Source: CAD feature listing. Evaluate the final solid. Frame: model axes, mm. A direction names the side the tool comes from. Round coordinates to 2 decimals unless told otherwise and drop trailing zeros. Write each loop counter-clockwise with the first axis right and the second up, starting at its lowest first coordinate (ties: lowest second). Pieces come first, ordered by that corner, then holes. Notation, with made-up numbers: M -33.75,41 L -5.75,41 A17 cw -5.75,58 Z; hole C -35,-25 d3. An arc over 180 degrees is marked long. Answer in a Markdown table with one row per item.
from build123d import *

# Parameters (mm, degrees)
CHAMFER_1_SIZE           = 2
CHAMFER_2_SIZE           = 1
PATTERN_CIRCULAR_1_COUNT = 6


with BuildPart() as part:
    # Эскиз1 → Повернуть1 (revolve)
    with BuildSketch(Plane.XY, mode=Mode.PRIVATE) as revolve_1_sk:
        Polygon((-118.03030303, 150), (11.96969697, 150), (11.96969697, 160), (-93.03030303, 160), (-93.03030303, 190), (-118.03030303, 190), align=None)
    revolve(revolve_1_sk.sketch.rotate(Axis((-311.484848485, 0, 0), (1, 0, 0)), 90), axis=Axis((-311.484848485, 0, 0), (1, 0, 0)))

    # Фаска1
    chamfer_1_edges = [part.edges().sort_by_distance(p)[0] for p in [
        (-93.03030303, 0, -190),
    ]]
    chamfer(chamfer_1_edges, length=CHAMFER_1_SIZE)

    # Фаска2
    chamfer_2_edges = [part.edges().sort_by_distance(p)[0] for p in [
        (-118.03030303, 0, -150),
    ]]
    chamfer(chamfer_2_edges, length=CHAMFER_2_SIZE)

    # Эскиз6 → Отверстие обработанное метчиком M121 (revolve, cut)
    with BuildSketch(Plane(origin=(-118.03030303, 172.5, 0), x_dir=(0, 0, 1), z_dir=(0, 1, 0))):
        Polygon((0, 0), (0, 35.814389157), (5.1, 32.75), (5.1, 0), align=None)
    hole_wizard_m121 = revolve(axis=Axis((-124.38030303, 172.5, 0), (1, 0, 0)), mode=Mode.SUBTRACT)

    # Круговой массив1: Отверстие обработанное метчиком M121 ×6 about axis
    pattern_circular_1_axis = Axis((0, 0, 0), (1, 0, 0))
    for i in range(1, PATTERN_CIRCULAR_1_COUNT):
        add(hole_wizard_m121.rotate(pattern_circular_1_axis, i * 360 / PATTERN_CIRCULAR_1_COUNT), mode=Mode.SUBTRACT)


solid = part.part
Q1. Section C-C (x = -48). Return loops of the section in (y, z), and give its area (3 significant figures).
Solutions:
| item | result |
|---|---|
| outline | C 0,0 d320; hole C 0,0 d300 |
| area | 9,740 mm2 |
Q2. Contact query for flat-ended pins moving along their axis: pin 1 Ø9 at (y, z) = (86.25, 149.39) entering from +X; pin 2 Ø13.5 at (y, z) = (172.5, 0) entering from +X; pin 3 Ø8 at (x, z) = (-8, -35.5) entering from +Y; pin 4 Ø12 at (x, z) = (-62.5, 36) entering from -Y. Output: stop coordinate, or through.
Solutions:
| item | result |
|---|---|
| pin 1 | passes through |
| pin 2 | stops at x = -93.03 |
| pin 3 | stops at y = 156.87 |
| pin 4 | stops at y = -157.16 |
Q3. Access query for faces 4 (the flat face through (-93.03, 138, 84)), 5 (the cylindrical face through (-106.69, 185.48, -41.19)). Directions: +Z, -Z, +X, -X, +Y, -Y. A direction counts if a zero-diameter tool reaches every point of the face in a straight line with its end or side. Return the directions, or none.
Solutions:
| item | result |
|---|---|
| face 4 | +X |
| face 5 | +X, -X |
Q4. Pull-direction query (Z, two-part tool) for faces 1 (the conical face through (-93.155, -186.524, -24.49)), 2 (the cylindrical face through (-105.71, -90.55, 152.13)), 3 (the flat face through (11.97, -143, -47)); classes: pulls with the +Z half, pulls with the -Z half, needs draft (parallel to the pull), parting line crosses it, or undercut.
Solutions:
| item | result |
|---|---|
| face 1 | parting line crosses it |
| face 2 | undercut |
| face 3 | needs draft |
Q5. Material intervals for probe 1 along Y at (x, z) = (-110.25, 0); probe 2 along Y at (x, z) = (-27, 0); probe 3 along Y at (x, z) = (-28.5, -4.5), sorted ascending.
Solutions:
| item | result |
|---|---|
| probe 1 | y = -190 to -177.6, -167.4 to -150, 150 to 167.4, 177.6 to 190 |
| probe 2 | y = -160 to -150, 150 to 160 |
| probe 3 | y = -159.94 to -149.93, 149.93 to 159.94 |
Q6. Section B-B (x = -106.5). Return loops of the section in (y, z), and give its area (3 significant figures).
Solutions:
| item | result |
|---|---|
| outline | C 0,0 d380; hole C -172.5,0 d10.2; hole C 0,0 d300; hole C -86.25,-149.39 d10.2; hole C -86.25,149.39 d10.2; hole C 86.25,-149.39 d10.2; hole C 86.25,149.39 d10.2; hole C 172.5,0 d10.2 |
| area | 42,200 mm2 |
Q7. Section A-A (y = 0). Return loops of the section in (x, z).
Solutions:
| item | result |
|---|---|
| outline | M -118.03,-190 L -95.03,-190 L -93.03,-188 L -93.03,-160 L 11.97,-160 L 11.97,-150 L -117.03,-150 L -118.03,-151 Z; M -118.03,151 L -117.03,150 L 11.97,150 L 11.97,160 L -93.03,160 L -93.03,188 L -95.03,190 L -118.03,190 Z |
